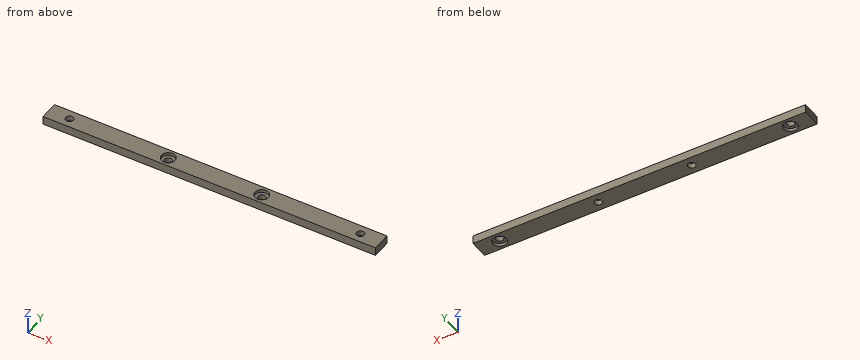
from build123d import *

# Parameters (mm, degrees)
SKETCH_1_W          = 60
SKETCH_1_H          = 10
SKETCH_1_R          = 1.8
EXTRUDE_1_DEPTH     = 4
SKETCH_2_R          = 3
CUT_EXTRUDE_1_DEPTH = 2
SKETCH_6_W          = 160
SKETCH_6_H          = 9
EXTRUDE_3_DEPTH     = 4
SKETCH_7_R          = 1.8
CUT_EXTRUDE_4_DEPTH = 4
SKETCH_8_R          = 3.25
CUT_EXTRUDE_5_DEPTH = 1.5
CUT_EXTRUDE_6_REACH = 113.7
SKETCH_9_R          = 1.8
CUT_EXTRUDE_7_REACH = 113.7
SKETCH_10_W         = 60
SKETCH_10_H         = 10
SKETCH_11_R         = 3.25
CUT_EXTRUDE_8_DEPTH = 1.5


with BuildPart() as part:
    # 草图1 → 凸台-拉伸1 (new body)
    with BuildSketch(Plane.XY):
        with Locations((30, 5)):
            Rectangle(SKETCH_1_W, SKETCH_1_H)
        with Locations((7.5, 5)):
            Circle(SKETCH_1_R, mode=Mode.SUBTRACT)
        with Locations((52.5, 5)):
            Circle(SKETCH_1_R, mode=Mode.SUBTRACT)
    extrude(amount=EXTRUDE_1_DEPTH)

    # 草图2 → 切除-拉伸1 (cut)
    with BuildSketch(Plane.XY.offset(4)):
        with Locations((7.5, 5)):
            Circle(SKETCH_2_R)
        with Locations((52.5, 5)):
            Circle(SKETCH_2_R)
    extrude(amount=-CUT_EXTRUDE_1_DEPTH, mode=Mode.SUBTRACT)

    # 草图6 → 凸台-拉伸3 (add)
    with BuildSketch(Plane.XY.offset(4)):
        with Locations((30, 14.5)):
            Rectangle(SKETCH_6_W, SKETCH_6_H)
    extrude(amount=-EXTRUDE_3_DEPTH)

    # 草图7 → 切除-拉伸4 (cut)
    with BuildSketch(Plane.XY.offset(4)):
        with Locations((-40, 14.5)):
            Circle(SKETCH_7_R)
        with Locations((100, 14.5)):
            Circle(SKETCH_7_R)
    extrude(amount=-CUT_EXTRUDE_4_DEPTH, mode=Mode.SUBTRACT)

    # 草图8 → 切除-拉伸5 (cut)
    with BuildSketch(Plane(origin=(0, 0, 0), x_dir=(-1, 0, 0), z_dir=(0, 0, -1))):
        with Locations((-100, 14.5)):
            Circle(SKETCH_8_R)
        with Locations((40, 14.5)):
            Circle(SKETCH_8_R)
    extrude(amount=-CUT_EXTRUDE_5_DEPTH, mode=Mode.SUBTRACT)

    # 草图9 → 切除-拉伸6 (cut, up to next)
    with BuildSketch(Plane.XY.offset(4), mode=Mode.PRIVATE) as cut_extrude_6_sk1:
        with Locations((7.5, 14.5)):
            Circle(SKETCH_9_R)
    cut_extrude_6_tool1 = extrude(cut_extrude_6_sk1.sketch, amount=-CUT_EXTRUDE_6_REACH, mode=Mode.PRIVATE) & part.part
    # 草图9 → 切除-拉伸6 (cut, up to next)
    with BuildSketch(Plane.XY.offset(4), mode=Mode.PRIVATE) as cut_extrude_6_sk2:
        with Locations((52.5, 14.5)):
            Circle(SKETCH_9_R)
    cut_extrude_6_tool2 = extrude(cut_extrude_6_sk2.sketch, amount=-CUT_EXTRUDE_6_REACH, mode=Mode.PRIVATE) & part.part
    add(cut_extrude_6_tool1.solids().sort_by_distance((7.5, 14.5, 4))[0], mode=Mode.SUBTRACT)
    add(cut_extrude_6_tool2.solids().sort_by_distance((52.5, 14.5, 4))[0], mode=Mode.SUBTRACT)

    # 草图10 → 切除-拉伸7 (cut, up to next)
    with BuildSketch(Plane.XY.offset(4), mode=Mode.PRIVATE) as cut_extrude_7_sk1:
        with Locations((30, 5)):
            Rectangle(SKETCH_10_W, SKETCH_10_H)
    cut_extrude_7_tool1 = extrude(cut_extrude_7_sk1.sketch, amount=-CUT_EXTRUDE_7_REACH, mode=Mode.PRIVATE) & part.part
    add(cut_extrude_7_tool1.solids().sort_by_distance((30, 5, 4))[0], mode=Mode.SUBTRACT)

    # 草图11 → 切除-拉伸8 (cut)
    with BuildSketch(Plane.XY.offset(4)):
        with Locations((7.5, 14.5)):
            Circle(SKETCH_11_R)
        with Locations((52.5, 14.5)):
            Circle(SKETCH_11_R)
    extrude(amount=-CUT_EXTRUDE_8_DEPTH, mode=Mode.SUBTRACT)


solid = part.part
Verification items for the finished model (mm, model axes). Give positions to 0.01 mm unless a question says otherwise; leave off trailing zeros. Loops run counter-clockwise (first coordinate to the right, second up) from the corner with the lowest first, then second, coordinate; pieces in that order, holes last.
1. Material ranges on probe 1 along Y at (x, z) = (100, 0.45); probe 2 along X at (y, z) = (12.25, 2.95); probe 3 along Z at (x, y) = (-42, 16.25), recorded low to high.
Derived:
probe 1: y = 10 to 11.25, 17.75 to 19
probe 2: x = -50 to 5.15, 9.85 to 50.15, 54.85 to 110
probe 3: z = 1.5 to 4
2. Cross-section at C-C on y = 14.5. Count the separate pieces of the cut face and the enclosed holes in it, and give its area (3 significant figures).
Derived:
separate pieces: 5
enclosed holes: 0
area: 565 mm2
3. Go/stop test with flat-tipped pins: P1, Ø1.5, axis at x = 51, y = 13.5, coming from the -Z side; P2, Ø4.5, axis at x = 7.5, y = 14.5, coming from the +Z side. Record where each tip stops, or that it passes through.
Derived:
P1: stops at z = 0
P2: stops at z = 2.5
4. Cross-section at B-B on z = 0.7. Record the cut outline in (x, y).
Derived:
outline: (-50, 10) - (110, 10) - (110, 19) - (-50, 19) - close; hole circle Ø6.5 at (-40, 14.5); hole circle Ø3.6 at (7.5, 14.5); hole circle Ø3.6 at (52.5, 14.5); hole circle Ø6.5 at (100, 14.5)
5. Cross-section at A-A on x = 7.5. Record the cut outline in (y, z).
Derived:
outline: (10, 0) - (12.7, 0) - (12.7, 2.5) - (11.25, 2.5) - (11.25, 4) - (10, 4) - close; (16.3, 0) - (19, 0) - (19, 4) - (17.75, 4) - (17.75, 2.5) - (16.3, 2.5) - close
